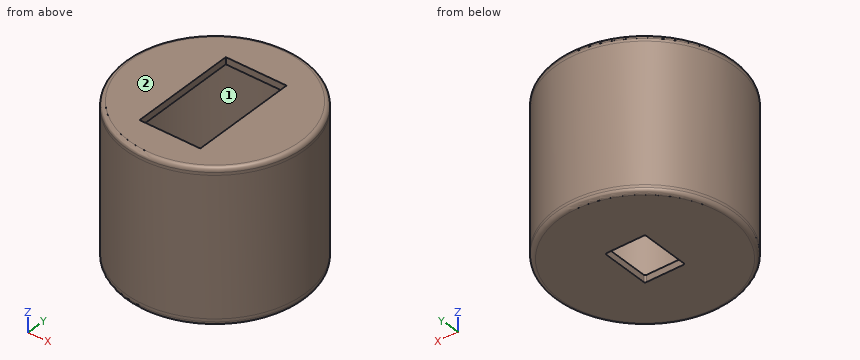
```python
from build123d import *

# Parameters (mm, degrees)
SKETCH1_R           = 6.5
SKETCH1_R_2         = 6
BOSS_EXTRUDE1_DEPTH = 10
BOSS_EXTRUDE2_START = 0.5
SKETCH2_R           = 6.5
BOSS_EXTRUDE2_DEPTH = 0.5
SKETCH3_R           = 6.5
SKETCH3_W           = 4.4
SKETCH3_H           = 7.8
BOSS_EXTRUDE3_DEPTH = 0.5
SKETCH4_W           = 2.9
SKETCH4_H           = 3.6
CUT_EXTRUDE1_DEPTH  = 1
FILLET1_R           = 0.1
FILLET2_R           = 0.3


with BuildPart() as part:
    # Sketch1 → Boss-Extrude1 (new body)
    with BuildSketch(Plane.XY):
        Circle(SKETCH1_R)
        Circle(SKETCH1_R_2, mode=Mode.SUBTRACT)
    extrude(amount=BOSS_EXTRUDE1_DEPTH)

    # Sketch2 → Boss-Extrude2 (add)
    with BuildSketch(Plane(origin=(0, 0, 0), x_dir=(-1, 0, 0), z_dir=(0, 0, -1)).offset(BOSS_EXTRUDE2_START)):
        Circle(SKETCH2_R)
    extrude(amount=-BOSS_EXTRUDE2_DEPTH)

    # Sketch3 → Boss-Extrude3 (add)
    with BuildSketch(Plane.XY.offset(10)):
        with Locations(Location((0, 0, 0), (0, 0, 180))):
            Circle(SKETCH3_R)
        with Locations((0.018144407, -0.2)):
            Rectangle(SKETCH3_W, SKETCH3_H, mode=Mode.SUBTRACT)
    extrude(amount=BOSS_EXTRUDE3_DEPTH)

    # Sketch4 → Cut-Extrude1 (cut)
    with BuildSketch(Plane(origin=(0, 0, -0.5), x_dir=(-1, 0, 0), z_dir=(0, 0, -1))):
        Rectangle(SKETCH4_W, SKETCH4_H)
    extrude(amount=-CUT_EXTRUDE1_DEPTH, mode=Mode.SUBTRACT)

    # Fillet1
    fillet1_edges = [part.edges().sort_by_distance(p)[0] for p in [
        (-1.45, 1.8, -0.25),
        (-1.45, -1.8, -0.25),
        (1.45, -1.8, -0.25),
        (1.45, 1.8, -0.25),
    ]]
    fillet(fillet1_edges, radius=FILLET1_R)

    # Fillet2
    fillet2_edges = [part.edges().sort_by_distance(p)[0] for p in [
        (6.5, 0, -0.5),
        (6.5, 0, 10.5),
    ]]
    fillet(fillet2_edges, radius=FILLET2_R)


solid = part.part
```
Read the model definition and answer for the solid it produces. Units are mm, in the model's axes. Face numbers are marked on the shaded views. Give positions to 0.01 mm unless a question says otherwise; leave off trailing zeros. Write each loop counter-clockwise with the first axis right and the second up, starting at its lowest first coordinate (ties: lowest second). Pieces come first, ordered by that corner, then holes. Notation, with made-up numbers: (76, 0.5) - (129, 0.5) arc R24 ccw to (129, 30.5) - close; hole circle Ø10 at (4.25, 74). An arc over 180 degrees is marked (long way). Write item = value, one per line. Start each with the question number.
Item 1: The mould has two halves that part along X. Classify the marked faces 1 and 2: +X half, -X half, draft (parallel to the pull), parting line (faces both ways), or undercut.
Item 2: Find section A-A (y = 0). Give the vertices of the cut face in (x, z), then the cut area to 3 significant figures.
Item 3: Find the intervals of material crossed by probe 1 along Z at (x, y) = (-2, -4.75); probe 2 along Y at (x, z) = (0, 6.75); probe 3 along X at (y, z) = (1, 4), in increasing order. Write a range as [from, to].
Item 4: Find section C-C (z = 6.5). Give the vertices of the cut face in (x, y), then the cut area to 3 significant figures.
Item 5: Each of these flat-tipped pins is pushed along its axis until it touches: P1, Ø4, axis at y = -4.5, z = 3.5, coming from the -X side; P2, Ø2, axis at x = 4.5, z = 1, coming from the +Y side; P3, Ø1.5, axis at x = 3, z = 3, coming from the +Y side. Where does it stop, or does it pass through?
Item 6: Find section B-B (x = 0). Give the vertices of the cut face in (y, z).
Response:
q1.face_1 = undercut
q1.face_2 = draft
q2.outline = (-6.5, -0.2) arc R0.3 ccw to (-6.2, -0.5) - (-1.45, -0.5) - (-1.45, 0) - (-6, 0) - (-6, 10) - (-2.18, 10) - (-2.18, 10.5) - (-6.2, 10.5) arc R0.3 ccw to (-6.5, 10.2) - close; (1.45, -0.5) - (6.2, -0.5) arc R0.3 ccw to (6.5, -0.2) - (6.5, 10.2) arc R0.3 ccw to (6.2, 10.5) - (2.22, 10.5) - (2.22, 10) - (6, 10) - (6, 0) - (1.45, 0) - close
q2.area = 19.3 mm²
q3.probe_1 = [-0.5, 0], [10, 10.5]
q3.probe_2 = [-6.5, -6], [6, 6.5]
q3.probe_3 = [-6.42, -5.92], [5.92, 6.42]
q4.outline = circle Ø13 at (0, 0); hole circle Ø12 at (0, 0)
q4.area = 19.6 mm²
q5.P1 = -6
q5.P2 = 5.48
q5.P3 = 6.1
q6.outline = (-6.5, -0.2) arc R0.3 ccw to (-6.2, -0.5) - (-1.8, -0.5) - (-1.8, 0) - (-6, 0) - (-6, 10) - (-4.1, 10) - (-4.1, 10.5) - (-6.2, 10.5) arc R0.3 ccw to (-6.5, 10.2) - close; (1.8, -0.5) - (6.2, -0.5) arc R0.3 ccw to (6.5, -0.2) - (6.5, 10.2) arc R0.3 ccw to (6.2, 10.5) - (3.7, 10.5) - (3.7, 10) - (6, 10) - (6, 0) - (1.8, 0) - close
